Model file for the job. Use its own axes, mm. A direction names the side the tool comes from. Round coordinates to 2 decimals unless told otherwise and drop trailing zeros. Order: outer loops, then holes, each group sorted by start corner. A loop starts at its lowest first (then second) coordinate and runs counter-clockwise, first axis right, second up. Notation, with made-up numbers: (-12, 81.5) - (3, 81.5) arc R20 cw to (3, 89.5) - close; hole circle Ø5 at (77.5, 19). An arc over 180 degrees is marked (long way). Put each result on its own line as item: value. Start each with the question number.
Item 1: Saw through at D-D on y = -8.75. List the corners of the cut face in (x, z).
Item 2: Saw through at C-C on z = 1.1. List the corners of the cut face in (x, y), plus the area to 3 significant figures.
Item 3: Which spindle directions (+Z, -Z, +X, -X, +Y, -Y) get a long thin tool onto all of the face, cutting with end or side? Do faces 4 (the face through (-1.2, 12, 1)), 5 (the face through (9.41, -6.82, 1.01)), 6 (the face through (5.4, -5.5, 2)), 7 (the face through (-9.387, -6.805, 1.014)), 8 (the face through (-10.61, -4.74, 1.01)). Say none if no direction does.
Item 4: Saw through at A-A on x = 0. List the corners of the cut face in (y, z), plus the area to 3 significant figures.
Item 5: Mould opens along X. For faces 1 (the face through (0.17, -12.65, 0.99)), 2 (the face through (1.2, 12, 1)), 3 (the face through (-11.039, 6.178, 0.986)) say: pulls with the +X half, pulls with the -X half, needs draft (parallel to the pull), parting line crosses it, or undercut.
Item 6: Pin check, flat tips, straight feed: pin 1 Ø0.6 at (y, z) = (12, 0.5) entering from +X; pin 2 Ø1.5 at (x, y) = (-6.5, -3) entering from -Z. Stop position of each tip, or through.
Item 7: Saw through at B-B on y = 0. List the corners of the cut face in (x, z), plus the area to 3 significant figures.
Item 8: Probe probe 1 along Y at (x, z) = (0, 1.45); probe 2 along Y at (x, z) = (0.5, 1.25); probe 3 along X at (y, z) = (11.5, 0.45). List the from-to ranges inside material, lowest first.
Autodesk Inventor part; units mm, degrees
ref_plane "YZ Plane" through (0, 0, 0) normal (1, 0, 0) x (0, 1, 0)
ref_plane "XZ Plane" through (0, 0, 0) normal (0, 1, 0) x (-1, 0, 0)
ref_plane "XY Plane" through (0, 0, 0) normal (0, 0, 1) x (1, 0, 0)
sketch "Skizze1" plane through (0, 0, 0) normal (0, 0, 1) x (1, 0, 0)
  circle A0 centre (0, 0) radius 12.65
  circle A1 centre (0, 0) radius 7.5
  dimension "d0" = 15
  dimension "d1" = 25.3
extrude "Extrusion1" add sketch "Skizze1" along normal blind 2
sketch "Skizze2" plane through (0, 0, 2) normal (0, 0, 1) x (1, 0, 0)
  circle A0 centre (0, 0) radius 12.65
  circle A1 centre (0, 0) radius 7.5
  arc A2 (-1.2, 10.5) -> (1.2, 10.5) centre (0, 10.5) ccw
  line L0 (-1.2, 10.5) -> (-1.2, 13.3719)
  line L1 (-1.2, 13.3719) -> (1.2, 13.3719)
  line L2 (1.2, 13.3719) -> (1.2, 10.5)
  line L3 (0, 12.65) -> (0, 7.5)
  line L4 (0, -17.8544) -> (0, 18.5762)
  dimension "d4" = 2.4
  dimension "d10" = 10.5
extrude "Extrusion2" cut sketch "Skizze2" against normal blind 2.4 contours L2 A2 L3 A0 | A0 L4 L1 L2 | L3 A2 L0 A0 | A0 L0 L1 L4
pattern_circular "Runde Anordnung1" count 3 over 360 about axis through (0, 0, 0) along (0, 0, 1) of "Extrusion2"
equation "\"d5\" = d4"
properties part number "P_Lagerschale_Deckel"
Results found:
1. outline: (-9.14, 0) - (9.14, 0) - (9.14, 2) - (-9.14, 2) - close
2. outline: (-11.51, -5.26) - (-9.69, -4.21) arc R1.2 cw to (-8.49, -6.29) - (-10.31, -7.34) arc R12.65 ccw to (10.31, -7.34) - (8.49, -6.29) arc R1.2 cw to (9.69, -4.21) - (11.51, -5.26) arc R12.65 ccw to (1.2, 12.59) - (1.2, 10.5) arc R1.2 cw to (-1.2, 10.5) - (-1.2, 12.59) arc R12.65 ccw to start; hole circle Ø15 at (0, 0)
2. area: 304 mm²
3. face 4: +Z, -Z, +Y
3. face 5: +Z, -Z, +X
3. face 6: +Z, +X, -X, +Y, -Y
3. face 7: +Z, -Z, -X
3. face 8: +Z, -Z
4. outline: (-12.65, 0) - (-7.5, 0) - (-7.5, 2) - (-12.65, 2) - close; (7.5, 0) - (9.3, 0) - (9.3, 2) - (7.5, 2) - close
4. area: 13.9 mm²
5. face 1: parting line crosses it
5. face 2: undercut
5. face 3: pulls with the -X half
6. pin 1: stops at x = 4.81
6. pin 2: stops at z = 0
7. outline: (-12.65, 0) - (-7.5, 0) - (-7.5, 2) - (-12.65, 2) - close; (7.5, 0) - (12.65, 0) - (12.65, 2) - (7.5, 2) - close
7. area: 20.6 mm²
8. probe 1: y = -12.65 to -7.5, 7.5 to 9.3
8. probe 2: y = -12.64 to -7.48, 7.48 to 9.41
8. probe 3: x = -5.27 to -1.2, 1.2 to 5.27
